Input: part model. Units: mm. Frame: model coordinates. A direction names the side the tool comes from. Round coordinates to 2 decimals unless told otherwise and drop trailing zeros. Write each loop counter-clockwise with the first axis right and the second up, starting at its lowest first coordinate (ties: lowest second). Pieces come first, ordered by that corner, then holes. Notation, with made-up numbers: (-21, 65.5) -> (3, 65.5) arc R13 ccw to (3, 71.5) -> close; hole circle Ø8 at (2.5, -27). An arc over 180 degrees is marked (long way). Use CSV: the item, a comma, the result in double quotes.
```python
from build123d import *

# Parameters (mm, degrees)
SKETCH1_R           = 2
BOSS_EXTRUDE1_DEPTH = 8
CUT_EXTRUDE1_DEPTH  = 5


with BuildPart() as part:
    # Sketch1 → Boss-Extrude1 (new body)
    with BuildSketch(Plane(origin=(0, 0, 0), x_dir=(1, 0, 0), z_dir=(0, 1, 0))):
        with BuildLine():
            Line((121.34297014, 11.1299482), (86.34297014, 11.1299482))
            Line((86.34297014, 11.1299482), (-63.65702986, 8.6299482))
            ThreePointArc((-63.65702986, 8.6299482), (-68.65702986, 3.6299482), (-63.65702986, -1.3700518))
            Line((-63.65702986, -1.3700518), (86.34297014, -3.8700518))
            ThreePointArc((86.34297014, -3.8700518), (89.524950656, -3.161590654), (92.105781954, -1.1700518))
            ThreePointArc((92.105781954, -1.1700518), (93.826336153, 0.157640769), (95.947656497, 0.6299482))
            Line((95.947656497, 0.6299482), (111.738283784, 0.6299482))
            ThreePointArc((111.738283784, 0.6299482), (113.859604128, 0.157640769), (115.580158327, -1.1700518))
            ThreePointArc((115.580158327, -1.1700518), (118.160989625, -3.161590654), (121.34297014, -3.8700518))
            ThreePointArc((121.34297014, -3.8700518), (125.450889322, -2.645001999), (128.216833683, 0.6299482))
            ThreePointArc((128.216833683, 0.6299482), (127.617920339, 7.737867381), (121.34297014, 11.1299482))
        make_face()
        with Locations(Location((-63.65702986, 3.6299482, 0), (0, 0, 270))):
            Circle(SKETCH1_R, mode=Mode.SUBTRACT)
        with Locations(Location((86.34297014, 3.6299482, 0), (0, 0, 270))):
            Circle(SKETCH1_R, mode=Mode.SUBTRACT)
        with Locations(Location((121.34297014, 3.6299482, 0), (0, 0, 270))):
            Circle(SKETCH1_R, mode=Mode.SUBTRACT)
    extrude(amount=BOSS_EXTRUDE1_DEPTH)

    # Sketch2 → Cut-Extrude1 (cut)
    with BuildSketch(Plane(origin=(0, 8, 0), x_dir=(1, 0, 0), z_dir=(0, 1, 0))):
        with BuildLine():
            Line((-53.693130943, 5.796013182), (5.024715148, 6.77464395))
            ThreePointArc((5.024715148, 6.77464395), (8.222259227, 3.6299482), (5.024715148, 0.48525245))
            Line((5.024715148, 0.48525245), (-53.693130943, 1.463883218))
            ThreePointArc((-53.693130943, 1.463883218), (-55.823395663, 3.6299482), (-53.693130943, 5.796013182))
        make_face()
        with BuildLine():
            Line((96.34297014, 8.3799482), (111.599382505, 8.3799482))
            ThreePointArc((111.599382505, 8.3799482), (114.099382505, 5.8799482), (111.599382505, 3.3799482))
            Line((111.599382505, 3.3799482), (96.34297014, 3.3799482))
            ThreePointArc((96.34297014, 3.3799482), (93.84297014, 5.8799482), (96.34297014, 8.3799482))
        make_face()
        with BuildLine():
            Line((15.021938142, 6.941264333), (76.270767974, 7.962078164))
            ThreePointArc((76.270767974, 7.962078164), (80.675701747, 3.6299482), (76.270767974, -0.702181764))
            Line((76.270767974, -0.702181764), (15.021938142, 0.318632067))
            ThreePointArc((15.021938142, 0.318632067), (11.765350737, 3.6299482), (15.021938142, 6.941264333))
        make_face()
    extrude(amount=-CUT_EXTRUDE1_DEPTH, mode=Mode.SUBTRACT)


solid = part.part
```
Item 1: Section query A-A on y = 1.25. Return the cut outline in (x, z), plus the area to 3 significant figures.
Worked answers:
outline,"(-63.66, -8.63) -> (86.34, -11.13) -> (121.34, -11.13) arc R7.5 ccw (long way) to (115.58, 1.17) arc R5 cw to (111.74, -0.63) -> (95.95, -0.63) arc R5 cw to (92.11, 1.17) arc R7.5 ccw to (86.34, 3.87) -> (-63.66, 1.37) arc R5 ccw to start; hole circle Ø4 at (-63.66, -3.63); hole circle Ø4 at (86.34, -3.63); hole circle Ø4 at (121.34, -3.63)"
area,"2,380 mm²"
Item 2: Pull-direction query (X, two-part tool) for faces 4 (the face through (-68.656, 3.944, -3.74)), 5 (the face through (104, 4, -11.13)), 6 (the face through (113.83, 3.94, -0.17)); classes: +X half, -X half, draft (parallel to the pull), parting line (faces both ways), or undercut.
Worked answers:
face 4,"-X half"
face 5,"draft"
face 6,"undercut"
Item 3: First-contact query: pin 1 Ø4 at (y, z) = (2, -4.5) entering from -X; pin 2 Ø1.5 at (x, y) = (38.5, 5) entering from +Z; pin 3 Ø4 at (x, y) = (105.5, 4.5) entering from +Z; pin 4 Ø4 at (x, y) = (-25.5, 6) entering from -Z. Flat tips, straight axial feed; report the tip coordinate or a pass-through.
Worked answers:
pin 1,"stops at x = -68.66"
pin 2,"stops at z = 3.09"
pin 3,"stops at z = -0.63"
pin 4,"stops at z = -9.3"
Item 4: Section query B-B on x = -5. Return the cut outline in (y, z), plus the area to 3 significant figures.
Worked answers:
outline,"(0, -9.61) -> (8, -9.61) -> (8, -6.61) -> (3, -6.61) -> (3, -0.65) -> (8, -0.65) -> (8, 2.35) -> (0, 2.35) -> close"
area,"65.9 mm²"
Item 5: Set-up query: faces 1 (the face through (89.483, 3.944, 3.181)), 2 (the face through (114.1, 5.5, -5.9)), 3 (the face through (-61.674, 3.944, -3.89)). Return all of +Z, -Z, +X, -X, +Y, -Y with unobstructed straight access to the full face (end or side cutting, diameter ignored); none if empty.
Worked answers:
face 1,"+Z, +Y, -Y"
face 2,"+Y"
face 3,"+Y, -Y"
Item 6: Section query C-C on x = 22.5. Return the cut outline in (y, z), plus the area to 3 significant figures.
Worked answers:
outline,"(0, -10.07) -> (8, -10.07) -> (8, -7.07) -> (3, -7.07) -> (3, -0.19) -> (8, -0.19) -> (8, 2.81) -> (0, 2.81) -> close"
area,"68.6 mm²"
Item 7: Line query: line 1 (X direction, y = 2, z = -3.25); line 2 (X direction, y = 2.25, z = -2.25); line 3 (Y direction, x = 33, z = -1.5). Output: solid intervals per line, ascending.
Worked answers:
line 1,"x = -68.64 to -65.62, -61.69 to 84.38, 88.31 to 119.38, 123.31 to 128.83"
line 2,"x = -68.46 to -65.1, -62.21 to 84.9, 87.79 to 119.9, 122.79 to 128.71"
line 3,"y = 0 to 3"
